For this review, use the dimensioned drawing (mm, ordinates from the lowest corner) and the shaded views. A direction names the side the tool comes from. Coordinates: 2 decimals unless noted, no trailing zeros. Loops run counter-clockwise (first coordinate to the right, second up) from the corner with the lowest first, then second, coordinate; pieces in that order, holes last. Notation, with made-up numbers: M 43,7.25 L 60,7.25 A32 cw 60,34.25 Z; hole C 57.25,-3.5 d7. An arc over 180 degrees is marked long. One line per item, written item: value.
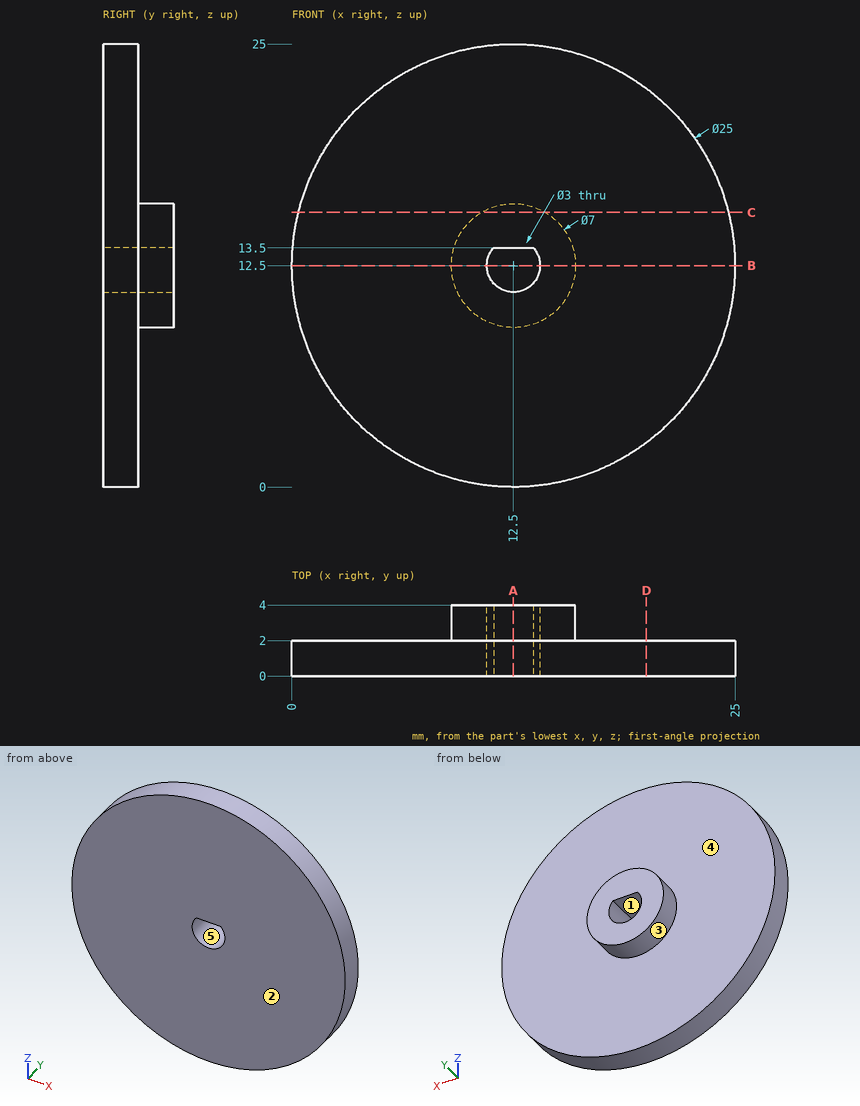
(1) Add section B-B on z = 12.5. State the section outline as (x, y) points, then the cut area to 3 significant figures.
Checks:
outline: M 0,0 L 11,0 L 11,4 L 9,4 L 9,2 L 0,2 Z; M 14,0 L 25,0 L 25,2 L 16,2 L 16,4 L 14,4 Z
area: 52.0 mm^2
(2) Draft analysis for pull direction Z (two halves, no side actions). For the marked faces 3, 4 and 5, state which applies: pulls with the +Z half, pulls with the -Z half, needs draft (parallel to the pull), parting line crosses it, or undercut.
Checks:
face 3: parting line crosses it
face 4: needs draft
face 5: undercut
(3) Tool access review of the marked faces 1 and 2: name each direction out of +Z, -Z, +X, -X, +Y, -Y from which nothing blocks a thin tool from reaching the whole face with its end or side.
Checks:
face 1: +Y, -Y
face 2: +Z, -Z, +X, -X, -Y
(4) Add section C-C on z = 15.5. State the section outline as (x, y) points.
Checks:
outline: M 0.37,0 L 24.63,0 L 24.63,2 L 14.3,2 L 14.3,4 L 10.7,4 L 10.7,2 L 0.37,2 Z
(5) Insertion check: pin 1 Ø4 at (x, z) = (21, 20) entering from +Y. The pin has a flat end and moves straight along its axis. Give the tip position at first contact, or say it passes through.
Checks:
pin 1: y = 2
(6) To check wall thickness, follow L1, parallel to X at y = 3, z = 12.5; L2, parallel to Z at x = 12.5, y = 1.6; L3, parallel to Y at x = 7, z = 14.25. State the ranges of each line that lie inside material, in increasing order. Write a range as [from, to].
Checks:
L1: [9, 11], [14, 16]
L2: [0, 11], [13.5, 25]
L3: [0, 2]
(7) Add section A-A on x = 12.5. State the section outline as (y, z) points, then the cut area to 3 significant figures.
Checks:
outline: M 0,0 L 2,0 L 2,9 L 4,9 L 4,11 L 0,11 Z; M 0,13.5 L 4,13.5 L 4,16 L 2,16 L 2,25 L 0,25 Z
area: 54.0 mm^2
(8) Add section D-D on x = 20. State the section outline as (y, z) points.
Checks:
outline: M 0,2.5 L 2,2.5 L 2,22.5 L 0,22.5 Z
